from build123d import *

# Parameters (mm, degrees)
SKETCH1_R           = 3.7
BOSS_EXTRUDE1_DEPTH = 2
SKETCH2_R           = 10
SKETCH2_R_2         = 3.8
BOSS_EXTRUDE2_DEPTH = 2
SKETCH4_W           = 12
SKETCH4_H           = 0.2
CUT_EXTRUDE1_DEPTH  = 4
FILLET3_R           = 0.35
FILLET4_R           = 0.15
FILLET6_R           = 2
BOSS_EXTRUDE6_DEPTH = 2
CIRPATTERN1_COUNT   = 5
SKETCH11_R          = 5
SKETCH11_R_2        = 4
BOSS_EXTRUDE7_DEPTH = 2
BOSS_EXTRUDE7_DRAFT = 3
FILLET10_R          = 0.2


with BuildPart() as part:
    # Sketch1 → Boss-Extrude1 (new body)
    with BuildSketch(Plane(origin=(0, 0, 0), x_dir=(1, 0, 0), z_dir=(0, 1, 0))):
        Polygon((-6, 6), (-6, -13.291502622), (-6, -19), (-2.70227506, -19), (-3.619175359, -13.8), (0, -13.8), (3.619175359, -13.8), (2.70227506, -19), (6, -19), (6, -13.291502622), (6, 6), align=None)
        with Locations(Location((0, 0, 0), (0, 0, 270))):
            Circle(SKETCH1_R, mode=Mode.SUBTRACT)
    extrude(amount=BOSS_EXTRUDE1_DEPTH)

    # Sketch2 → Boss-Extrude2 (add)
    with BuildSketch(Plane(origin=(0, 0, 0), x_dir=(1, 0, 0), z_dir=(0, 1, 0))):
        Circle(SKETCH2_R)
        Circle(SKETCH2_R_2, mode=Mode.SUBTRACT)
    extrude(amount=BOSS_EXTRUDE2_DEPTH)

    # Sketch4 → Cut-Extrude1 (cut)
    with BuildSketch(Plane(origin=(0, 2, 0), x_dir=(1, 0, 0), z_dir=(0, 1, 0))):
        with Locations((0, -18.9)):
            Rectangle(SKETCH4_W, SKETCH4_H)
    extrude(amount=-CUT_EXTRUDE1_DEPTH, mode=Mode.SUBTRACT)

    # Fillet3
    fillet3_edges = [part.edges().sort_by_distance(p)[0] for p in [
        (3.619175359, 1, 13.8),
        (-3.619175359, 1, 13.8),
    ]]
    fillet(fillet3_edges, radius=FILLET3_R)

    # Fillet4
    fillet4_edges = [part.edges().sort_by_distance(p)[0] for p in [
        (2.737540456, 1, 18.8),
        (-2.737540456, 1, 18.8),
    ]]
    fillet(fillet4_edges, radius=FILLET4_R)

    # Fillet6
    fillet6_edges = [part.edges().sort_by_distance(p)[0] for p in [
        (6, 1, 8),
        (-6, 1, 8),
    ]]
    fillet(fillet6_edges, radius=FILLET6_R)

    # Sketch8 → Boss-Extrude6 (add)
    with BuildSketch(Plane(origin=(0, 2, 0), x_dir=(1, 0, 0), z_dir=(0, 1, 0))):
        Polygon((-0.5, 3.65), (0, 2.65), (0.5, 3.65), (0.5, 4.15), (-0.5, 4.15), align=None)
    boss_extrude6 = extrude(amount=-BOSS_EXTRUDE6_DEPTH)

    # CirPattern1: Boss-Extrude6 ×5 about axis
    cirpattern1_axis = Axis((0, 0, 0), (0, 1, 0))
    for i in range(1, CIRPATTERN1_COUNT):
        add(boss_extrude6.rotate(cirpattern1_axis, i * 360 / CIRPATTERN1_COUNT))


with BuildPart() as boss_extrude7_tool:
    # Sketch11 → Boss-Extrude7 (with draft: the straight prism first)
    with BuildSketch(Plane(origin=(0, 2, 0), x_dir=(1, 0, 0), z_dir=(0, 1, 0))):
        Circle(SKETCH11_R)
        Circle(SKETCH11_R_2, mode=Mode.SUBTRACT)
    extrude(amount=BOSS_EXTRUDE7_DEPTH)
    # Boss-Extrude7: the draft: its side faces are tilted about the plane it starts from
    boss_extrude7_sides = [boss_extrude7_tool.faces().sort_by_distance(p)[0] for p in [
        (-5, 3, 0),
        (-4, 3, 0),
    ]]
    draft(boss_extrude7_sides, Plane(origin=(0, 2, 0), x_dir=(1, 0, 0), z_dir=(0, 1, 0)), BOSS_EXTRUDE7_DRAFT)


with BuildPart() as part_1:
    add(part.part)

    # Boss-Extrude7: add boss_extrude7_tool
    add(boss_extrude7_tool.part)

    # Fillet10
    fillet10_edges = [part_1.edges().sort_by_distance(p)[0] for p in [
        (0, 1, -2.65),
        (2.520299768, 1, -0.818895035),
        (1.557630919, 1, 2.143895035),
        (-1.557630919, 1, 2.143895035),
        (-2.520299768, 1, -0.818895035),
    ]]
    fillet(fillet10_edges, radius=FILLET10_R)


solid = part_1.part
For this review, take the finished solid that the model builds, in its own axes (mm). A direction names the side the tool comes from. Round coordinates to 2 decimals unless told otherwise and drop trailing zeros. Write each loop counter-clockwise with the first axis right and the second up, starting at its lowest first coordinate (ties: lowest second). Pieces come first, ordered by that corner, then holes. Notation, with made-up numbers: (-7, 58) - (29, 58) arc R6 ccw to (29, 66) - close; hole circle Ø9 at (31.25, 19.5). An arc over 180 degrees is marked (long way). Use a Markdown table: item, result.
Q1. Clearance check with flat-ended pins moving along their axes: pin 1 (2 mm diameter, centred on x = 0, y = 1, fed in from +Z); pin 2 (1.5 mm diameter, centred on x = 2.5, y = 2, fed in from -Z); pin 3 (1.6 mm diameter, centred on y = 1, z = 15.5, fed in from -X); pin 4 (6 mm diameter, centred on x = 2.5, z = 0.5, fed in from +Y). State where each tip first meets the part, or that it passes through.
Derived:
| item | result |
|---|---|
| pin 1 | stops at z = 13.8 |
| pin 2 | stops at z = -9.85 |
| pin 3 | stops at x = -6 |
| pin 4 | stops at y = 4 |
Q2. We need section C-C (z = 5.5). Give the boundary of the cut face in (x, y), plus the area to 3 significant figures.
Derived:
| item | result |
|---|---|
| outline | (-8.35, 0) - (8.35, 0) - (8.35, 2) - (-8.35, 2) - close |
| area | 33.4 mm2 |
Q3. The part is to be moulded in two halves that separate along X. For faces 5 (the conical face through (4.71, 3.21, -1.48)), 6 (the flat face through (-6, 1, 14)), 7 (the cylindrical face through (2.195, 0.986, -2.978)), say which applies: pulls with the +X half, pulls with the -X half, needs draft (parallel to the pull), parting line crosses it, or undercut.
Derived:
| item | result |
|---|---|
| face 5 | parting line crosses it |
| face 6 | pulls with the -X half |
| face 7 | undercut |
Q4. We need section B-B (x = 8.5). Give the boundary of the cut face in (y, z).
Derived:
| item | result |
|---|---|
| outline | (0, -5.27) - (2, -5.27) - (2, 5.27) - (0, 5.27) - close |
Q5. Wall thickness on line 1 along Y through (x, z) = (3.75, -5); line 2 along X through (y, z) = (1.7, 14.5); line 3 along Z through (x, y) = (1.75, 2.15): over which ranges is each line inside the solid? List them lowest first.
Derived:
| item | result |
|---|---|
| line 1 | y = 0 to 2 |
| line 2 | x = -6 to -3.5, 3.5 to 6 |
| line 3 | z = -4.68 to -3.61, 3.61 to 4.68 |
Q6. Machinability: for faces 1 (the flat face through (-3, 2, -1)), 2 (the flat face through (6, 1, 14)), 3 (the cylindrical face through (3.5, 1, 1.2)), 4 (the flat face through (-4, 1, 18.8)), which of the approach directions +Z, -Z, +X, -X, +Y, -Y give a long, thin tool a straight path to every point of the face, cutting with its end or side? Answer none if there is none.
Derived:
| item | result |
|---|---|
| face 1 | +Y |
| face 2 | +Z, +X, +Y, -Y |
| face 3 | +Y, -Y |
| face 4 | +Z, +X, -X, +Y, -Y |
Q7. We need section A-A (z = 0). Give the boundary of the cut face in (x, y), plus the area to 3 significant figures.
Derived:
| item | result |
|---|---|
| outline | (-10, 0) - (-3.7, 0) - (-3.7, 2) - (-4, 2) - (-4.1, 4) - (-4.9, 4) - (-5, 2) - (-10, 2) - close; (3.7, 0) - (10, 0) - (10, 2) - (5, 2) - (4.9, 4) - (4.1, 4) - (4, 2) - (3.7, 2) - close |
| area | 28.8 mm2 |
